```python
from build123d import *

# Parameters (mm, degrees)
BOX035_W          = 162
BOX035_H          = 3
BOX035_DEPTH      = 162
CYLINDER010_R     = 30
CYLINDER010_DEPTH = 31
CYLINDER011_R     = 37.5
CYLINDER011_DEPTH = 46
CYLINDER012_R     = 40
CYLINDER012_DEPTH = 18


with BuildPart() as cube030:
    # Box035 → Box035 (new body)
    with BuildSketch(Plane.XY):
        with Locations((81, 1.5)):
            Rectangle(BOX035_W, BOX035_H)
    extrude(amount=BOX035_DEPTH)


with BuildPart() as cylinder010:
    # Cylinder010 → Cylinder010 (new body)
    with BuildSketch(Plane(origin=(81, 2, 81), x_dir=(1, 0, 0), z_dir=(0, 1, 0))):
        Circle(CYLINDER010_R)
    extrude(amount=CYLINDER010_DEPTH)


with BuildPart() as cylinder011:
    # Cylinder011 → Cylinder011 (new body)
    with BuildSketch(Plane(origin=(81, -45, 81), x_dir=(1, 0, 0), z_dir=(0, 1, 0))):
        Circle(CYLINDER011_R)
    extrude(amount=CYLINDER011_DEPTH)


with BuildPart() as f_240mm:
    # Cylinder012 → Cylinder012 (new body)
    with BuildSketch(Plane(origin=(81, -17, 81), x_dir=(1, 0, 0), z_dir=(0, 1, 0))):
        Circle(CYLINDER012_R)
    extrude(amount=CYLINDER012_DEPTH)

    # Fusion008: union Cube030, Cylinder010, Cylinder011
    add(cube030.part)
    add(cylinder010.part)
    add(cylinder011.part)


with BuildPart() as f_240mm_1:
    # Fusion008 placement: moved
    add(f_240mm.part.moved(Location((4.5, -2, 3))))


solid = f_240mm_1.part
```
The model under review builds one solid part; all positions refer to its coordinate system, in mm. A direction names the side the tool comes from. Coordinates: 2 decimals unless noted, no trailing zeros. Order: outer loops, then holes, each group sorted by start corner. A loop starts at its lowest first (then second) coordinate and runs counter-clockwise, first axis right, second up. Notation, with made-up numbers: M 16,-28 L 60,-28 A28 cw 60,10 Z; hole C -8.75,35.25 d8. An arc over 180 degrees is marked long. One line per question, with ' | ' between items.
(1) Add section A-A, the plane x = 85.5. Write out the cut boundary in (y, z).
Geometry results:
outline: M -47,46.5 L -19,46.5 L -19,44 L -2,44 L -2,3 L 1,3 L 1,54 L 31,54 L 31,114 L 1,114 L 1,165 L -2,165 L -2,124 L -19,124 L -19,121.5 L -47,121.5 Z
(2) Insertion check: pin 1 (12 mm diameter, centred on x = 131, z = 22, fed in from -Y); pin 2 (6 mm diameter, centred on x = 88.5, y = 16.5, fed in from +Z); pin 3 (12 mm diameter, centred on y = 8, z = 98, fed in from +X). Each pin has a flat end and moves straight along its axis. Give the tip position at first contact, or say it passes through.
Geometry results:
pin 1: stops at y = -2 | pin 2: stops at z = 114 | pin 3: stops at x = 114.41
(3) For probe 1 along Y at (x, z) = (106.5, 132); probe 2 along Z at (x, y) = (87, -35); probe 3 along Z at (x, y) = (87, 4.5), list the stretches that pass through material, from the lowest coordinate up. Write a range as from..to.
Geometry results:
probe 1: y = -2..1 | probe 2: z = 46.53..121.47 | probe 3: z = 54.04..113.96
(4) Machinability: for faces 1 (the face through (97, -19, 48)), 2 (the face through (85, 31, 84)), 3 (the face through (63.389, 15.79, 63.725)), which of the approach directions +Z, -Z, +X, -X, +Y, -Y give a long, thin tool a straight path to every point of the face, cutting with its end or side? Answer none if there is none.
Geometry results:
face 1: -Y | face 2: +Z, -Z, +X, -X, +Y | face 3: +Y
(5) Add section B-B, the plane z = 84. Write out the cut boundary in (x, y), then the cut area to 3 significant figures.
Geometry results:
outline: M 4.5,-2 L 45.5,-2 L 45.5,-19 L 48,-19 L 48,-47 L 123,-47 L 123,-19 L 125.5,-19 L 125.5,-2 L 166.5,-2 L 166.5,1 L 115.5,1 L 115.5,31 L 55.5,31 L 55.5,1 L 4.5,1 Z | area: 5,750 mm²
(6) Add section C-C, the plane y = -34. Write out the cut boundary in (x, z).
Geometry results:
outline: C 85.5,84 d75
(7) Add section D-D, the plane z = 49.5. Write out the cut boundary in (x, y).
Geometry results:
outline: M 4.5,-2 L 65.26,-2 L 65.26,-19 L 70.8,-19 L 70.8,-47 L 100.2,-47 L 100.2,-19 L 105.74,-19 L 105.74,-2 L 166.5,-2 L 166.5,1 L 4.5,1 Z
